Geometry check sheet. Reference: the model listing, model coordinates, mm. Face numbers are marked on the shaded views. A direction names the side the tool comes from. Give positions to 0.01 mm unless a question says otherwise; leave off trailing zeros. Write each loop counter-clockwise with the first axis right and the second up, starting at its lowest first coordinate (ties: lowest second). Pieces come first, ordered by that corner, then holes.
(1) Cross-section at A-A (z = -52). Record the boundary of the cut face in (x, y).
(2) Mould release check, pull along Z, two halves, no side actions. Record for the marked faces 1, 2 and 3: +Z half, -Z half, draft (parallel to the pull), parting line (faces both ways), or undercut.
(3) Depth check by flat-ended pin: P1, Ø8, axis at x = -64.5, z = -32, coming from the +Y side. Enter the tip coordinate at first touch or a pass-through.
(4) Cross-section at B-B (y = 28.5). Record the boundary of the cut face in (x, z), and give its area (3 significant figures).
(5) Cross-section at C-C (x = -13.5). Record the boundary of the cut face in (y, z), and give its area (3 significant figures).
(6) Cross-section at D-D (x = -83). Record the boundary of the cut face in (y, z), and give its area (3 significant figures).
(7) Thickness scan on line 1 along X through (y, z) = (2.5, -66); line 2 along X through (y, z) = (8, -16.5); line 3 along Z through (x, y) = (-18.5, 10). Record the ranges inside material, lowest first.
(8) Tool access check on the marked faces 4 and 5. Record the directions out of +Z, -Z, +X, -X, +Y, -Y that give a thin tool (end or side, any length) a straight path to the whole face; none if there is none.
Autodesk Inventor part; units mm, degrees
ref_plane "YZ Plane" through (0, 0, 0) normal (1, 0, 0) x (0, 1, 0)
ref_plane "XZ Plane" through (0, 0, 0) normal (0, 1, 0) x (-1, 0, 0)
ref_plane "XY Plane" through (0, 0, 0) normal (0, 0, 1) x (1, 0, 0)
sketch "Sketch1" plane through (0, 0, 0) normal (0, 1, 0) x (-1, 0, 0)
  line L0 (0, 0) -> (105, 0)
  line L1 (105, 0) -> (105, -70)
  line L2 (105, -70) -> (0, -70)
  line L3 (0, -70) -> (0, 0)
  dimension "d0" = 105
  dimension "d1" = 70
extrude "Extrusion1" add sketch "Sketch1" along normal blind 4
sketch "Sketch2" plane through (0, 0, 0) normal (0, -1, 0) x (1, 0, 0)
  line L0 (-101.8, -3.2) -> (-84.8, -3.2)
  line L1 (-84.8, -3.2) -> (-84.8, -5.2)
  line L2 (-84.8, -5.2) -> (-99.8, -5.2)
  line L3 (-99.8, -5.2) -> (-99.8, -20.2)
  line L4 (-99.8, -20.2) -> (-101.8, -20.2)
  line L5 (-101.8, -20.2) -> (-101.8, -3.2)
  line L6 (-105, 0) -> (0, 0)
  line L7 (-105, -70) -> (-105, 0)
  line L8 (-52.5, 13.4533) -> (-52.5, -78.582) construction
  line L9 (-116.2226, -35) -> (14.8802, -35) construction
  line L10 (-3.2, -3.2) -> (-20.2, -3.2)
  line L11 (-20.2, -3.2) -> (-20.2, -5.2)
  line L12 (-20.2, -5.2) -> (-5.2, -5.2)
  line L13 (-5.2, -5.2) -> (-5.2, -20.2)
  line L14 (-5.2, -20.2) -> (-3.2, -20.2)
  line L15 (-3.2, -20.2) -> (-3.2, -3.2)
  line L16 (-101.8, -66.8) -> (-84.8, -66.8)
  line L17 (-84.8, -66.8) -> (-84.8, -64.8)
  line L18 (-84.8, -64.8) -> (-99.8, -64.8)
  line L19 (-99.8, -64.8) -> (-99.8, -49.8)
  line L20 (-99.8, -49.8) -> (-101.8, -49.8)
  line L21 (-101.8, -49.8) -> (-101.8, -66.8)
  line L22 (-3.2, -66.8) -> (-20.2, -66.8)
  line L23 (-3.2, -49.8) -> (-3.2, -66.8)
  line L24 (-5.2, -49.8) -> (-3.2, -49.8)
  line L25 (-5.2, -64.8) -> (-5.2, -49.8)
  line L26 (-20.2, -64.8) -> (-5.2, -64.8)
  line L27 (-20.2, -66.8) -> (-20.2, -64.8)
  dimension "d4" = 17
  dimension "d5" = 2
  dimension "d6" = 17
  dimension "d7" = 2
  dimension "d8" = 3.2
  dimension "d9" = 3.2
  dimension "d10" = 52.5
  dimension "d11" = 35
extrude "Extrusion2" cut sketch "Sketch2" against normal through all
sketch "Sketch3" plane through (0, 4, 0) normal (0, 1, 0) x (1, 0, 0)
  line L0 (-105, 70) -> (-105, 0)
  line L1 (-105, 70) -> (-105, 50)
  line L2 (-105, 50) -> (-102, 50)
  line L3 (-105, 70) -> (-85, 70)
  line L4 (0, 70) -> (-105, 70)
  line L5 (-85, 70) -> (-85, 67)
  line L6 (-85, 67) -> (-102, 67)
  line L7 (-102, 67) -> (-102, 50)
  line L8 (-52.5, 99.9312) -> (-52.5, -17.7346) construction
  line L9 (-124.2156, 35) -> (28.5486, 35) construction
  line L10 (0, 70) -> (0, 50)
  line L11 (0, 50) -> (-3, 50)
  line L12 (0, 70) -> (-20, 70)
  line L13 (-20, 70) -> (-20, 67)
  line L14 (-20, 67) -> (-3, 67)
  line L15 (-3, 67) -> (-3, 50)
  line L16 (19.2156, 35) -> (-133.5486, 35) construction
  line L17 (-105, 0) -> (-105, 20)
  line L18 (-105, 20) -> (-102, 20)
  line L19 (-105, 0) -> (-85, 0)
  line L20 (-85, 0) -> (-85, 3)
  line L21 (-85, 3) -> (-102, 3)
  line L22 (-102, 3) -> (-102, 20)
  line L23 (-52.5, -29.9312) -> (-52.5, 87.7346) construction
  line L24 (0, 0) -> (0, 20)
  line L25 (0, 20) -> (-3, 20)
  line L26 (0, 0) -> (-20, 0)
  line L27 (-20, 0) -> (-20, 3)
  line L28 (-20, 3) -> (-3, 3)
  line L29 (-3, 3) -> (-3, 20)
  point P0 (-105, 20)
  point P1 (-20, 70)
  point P2 (0.75, 3)
  point P3 (2, 8)
  point P4 (2, 62)
  point P5 (0.75, 67)
  dimension "d15" = 20
  dimension "d16" = 3
  dimension "d17" = 20
  dimension "d18" = 3
  dimension "d19" = 52.5
  dimension "d20" = 35
extrude "Extrusion3" add sketch "Sketch3" along normal blind 28
fillet "Fillet2" radius 10 8 edges at (-85, 4, -1.5) (-20, 4, -1.5) (-1.5, 4, -20) (-103.5, 4, -20) (-1.5, 4, -50) (-103.5, 4, -50) (-85, 4, -68.5) (-20, 4, -68.5)
properties part number "TestingPlatform_standardStack01"
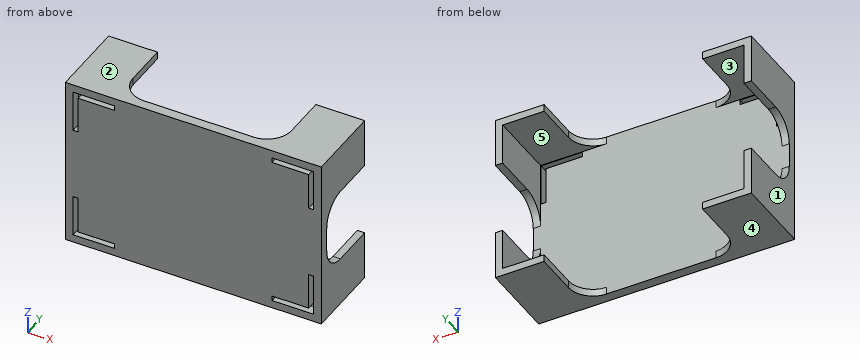
Reply:
1. outline: (-105, 0) - (-101.8, 0) - (-101.8, 4) - (-102, 4) - (-102, 32) - (-105, 32) - close; (-99.8, 0) - (-5.2, 0) - (-5.2, 4) - (-99.8, 4) - close; (-3.2, 0) - (0, 0) - (0, 32) - (-3, 32) - (-3, 4) - (-3.2, 4) - close
2. face 1: draft
2. face 2: +Z half
2. face 3: undercut
3. P1: stops at y = 4
4. outline: (-105, -70) - (-85, -70) - (-85, -67) - (-102, -67) - (-102, -50) - (-105, -50) - close; (-105, -20) - (-102, -20) - (-102, -3) - (-85, -3) - (-85, 0) - (-105, 0) - close; (-20, -70) - (0, -70) - (0, -50) - (-3, -50) - (-3, -67) - (-20, -67) - close; (-20, -3) - (-3, -3) - (-3, -20) - (0, -20) - (0, 0) - (-20, 0) - close
4. area: 444 mm2
5. outline: (0, -70) - (32, -70) - (32, -67) - (4, -67) - (4, -66.8) - (0, -66.8) - close; (0, -64.8) - (4, -64.8) - (4, -5.2) - (0, -5.2) - close; (0, -3.2) - (4, -3.2) - (4, -3) - (32, -3) - (32, 0) - (0, 0) - close
5. area: 432 mm2
6. outline: (0, -70) - (8, -70) - (8, -67) - (4, -67) - (4, -3) - (8, -3) - (8, 0) - (0, 0) - close
6. area: 304 mm2
7. line 1: x = -105 to -101.8, -84.8 to -20.2, -3.2 to 0
7. line 2: x = -105 to -102, -3 to 0
7. line 3: z = -70 to -67, -3 to 0
8. face 4: -Z, +X, -X, +Y, -Y
8. face 5: +Y
